Autodesk Inventor part; units mm, degrees
ref_plane "YZ Plane" through (0, 0, 0) normal (1, 0, 0) x (0, 1, 0)
ref_plane "XZ Plane" through (0, 0, 0) normal (0, 1, 0) x (-1, 0, 0)
ref_plane "XY Plane" through (0, 0, 0) normal (0, 0, 1) x (1, 0, 0)
sketch "Boceto2" plane through (0, 0, 0) normal (1, 0, 0) x (0, 1, 0)
  line L0 (0, 0) -> (200, 0)
  line L1 (200, 0) -> (200, -30)
  line L2 (200, -30) -> (0, -30)
  circle A0 centre (185, -15) radius 3.5
  line L3 (0, -12) -> (55, -12)
  line L4 (55, -12) -> (55, -18)
  line L5 (55, -18) -> (0, -18)
  line L6 (0, 0) -> (0, -12)
  line L7 (0, -30) -> (0, -18)
  point P0 (200, -15)
  dimension "d2" = 7
  dimension "d3" = 15
  dimension "d7" = 6
  dimension "d8" = 30
  dimension "d9" = 12
  dimension "d10" = 200
  dimension "d11" = 12
  dimension "d12" = 55
extrude "Extrusión1" add sketch "Boceto2" along normal blind 12
properties part number "ColumnaSoporte"
Geometry check sheet. Reference: the model listing, model coordinates, mm. A direction names the side the tool comes from. Round coordinates to 2 decimals unless told otherwise and drop trailing zeros. Loops run counter-clockwise (first coordinate to the right, second up) from the corner with the lowest first, then second, coordinate; pieces in that order, holes last. Notation, with made-up numbers: (42, -29.5) - (63, -29.5) arc R22 ccw to (63, 1.5) - close; hole circle Ø3 at (81.25, -28). An arc over 180 degrees is marked (long way). Answer as CSV lines item,"result".
(1) Cross-section at A-A, the plane y = 185. Enter the section's corners in (x, z).
Output values:
outline,"(0, -30) - (12, -30) - (12, -18.5) - (0, -18.5) - close; (0, -11.5) - (12, -11.5) - (12, 0) - (0, 0) - close"
(2) Cross-section at B-B, the plane z = -15. Enter the section's corners in (x, y), and give its area (3 significant figures).
Output values:
outline,"(0, 55) - (12, 55) - (12, 181.5) - (0, 181.5) - close; (0, 188.5) - (12, 188.5) - (12, 200) - (0, 200) - close"
area,"1,660 mm²"
(3) Set-up check for faces 4 (the face through (5.92, 188.34, -16.05)), 5 (the face through (6, 55, -15)): record each of +Z, -Z, +X, -X, +Y, -Y from which the full face is reachable in a straight line by a thin tool's end or side.
Output values:
face 4,"+X, -X"
face 5,"+X, -X, -Y"
(4) Material ranges on line 1 along Z through (x, y) = (3, 185); line 2 along Z through (x, y) = (11.25, 38), recorded low to high.
Output values:
line 1,"z = -30 to -18.5, -11.5 to 0"
line 2,"z = -30 to -18, -12 to 0"
(5) Release check for a two-part mould opening along Z. For faces 1 (the face through (6, 28, -18)), 2 (the face through (12, 99, -15)), 3 (the face through (6, 101, -30)) record: released by +Z, released by -Z, zero draft, split by the parting line, or undercut.
Output values:
face 1,"undercut"
face 2,"zero draft"
face 3,"released by -Z"
